Here's how the part is built. I have some questions about the finished solid (model axes, mm). A direction names the side the tool comes from. Give positions to 0.01 mm unless a question says otherwise; leave off trailing zeros. Loops run counter-clockwise (first coordinate to the right, second up) from the corner with the lowest first, then second, coordinate; pieces in that order, holes last.
Q1. I need wall thicknesses on line 1 (Y direction, x = 0, z = 5); line 2 (Z direction, x = 24, y = 40); line 3 (X direction, y = 9.5, z = 46). Which ranges of each line are inside material? Lowest first, please.
Q2. If we section it at B-B (z = 37.5): Please give me the cut outline in (x, y).
Q3. For faces 1 (the face through (3, 0, 0)), 2 (the face through (-2.75, -12.4, 25.04)), which set-ups out of +Z, -Z, +X, -X, +Y, -Y let a thin tool reach every point of the face, with its end or its side?
Q4. If we section it at C-C (x = 61): Please give me the cut outline in (y, z), plus the area to 3 significant figures.
Q5. If we section it at A-A (x = 8.5): Please give me the cut outline in (y, z), plus the area to 3 significant figures.
Q6. If we section it at D-D (x = 28): Please give me the cut outline in (y, z), plus the area to 3 significant figures.
Q7. Will these pins go through, and if not, where does the flat tip stop? P1, Ø10, axis at y = -5, z = 25, coming from the +X side; P2, Ø8, axis at x = -6, z = 33.5, coming from the +Y side; P3, Ø2, axis at x = -0.5, y = 0, coming from the -Z side; P4, Ø4, axis at x = 8, y = -45.5, coming from the -Z side.
from build123d import *

# Parameters (mm, degrees)
F0_R     = 12.7
F1_DEPTH = 50.8
F3_DEPTH = 2.54
F4_R     = 1.27
F5_DEPTH = 12.7


with BuildPart() as f1:
    # F0 (on Top) → F1 (new body)
    with BuildSketch(Plane.XY):
        Circle(F0_R)
    extrude(amount=F1_DEPTH)

    # F2 (on face) → F3 (join)
    with BuildSketch(Plane.XY.offset(50.8)):
        with BuildLine():
            Line((43.181052426, 26.7588622961), (25.5085228248, 43.9312561088))
            ThreePointArc((25.5085228248, 43.9312561088), (-43.9312561088, 25.5085228248), (-25.5085228248, -43.9312561088))
            Line((-25.5085228248, -43.9312561088), (-1.833987853, -50.7668837783))
            ThreePointArc((-1.833987853, -50.7668837783), (6.0769799698, -50.4352090751), (13.8403151675, -48.87827407))
            ThreePointArc((13.8403151675, -48.87827407), (5.917077838, -28.064349578), (10.982813992, -6.3771307669))
            ThreePointArc((10.982813992, -6.3771307669), (27.3066244447, 8.7731285653), (49.3108654889, 12.2097725094))
            ThreePointArc((49.3108654889, 12.2097725094), (46.8146101479, 19.7239011532), (43.181052426, 26.7588622961))
        make_face()
        with BuildLine():
            ThreePointArc((12.7, 0), (12.2631916257, -3.3021403894), (10.982813992, -6.3771307669))
            ThreePointArc((10.982813992, -6.3771307669), (-12.2631916257, 3.3021403894), (12.7, 0))
        make_face(mode=Mode.SUBTRACT)
        with BuildLine():
            ThreePointArc((63.0626482274, 7.4399192569), (56.4166545258, 10.4876551164), (49.3108654889, 12.2097725094))
            ThreePointArc((49.3108654889, 12.2097725094), (50.4263421578, 6.150123298), (50.8, 0))
            ThreePointArc((50.8, 0), (50.3191031963, -6.9733674448), (48.8855175779, -13.8147085071))
            ThreePointArc((48.8855175779, -13.8147085071), (54.5192002119, -18.4952896423), (56.6312561088, -25.5085228248))
            ThreePointArc((56.6312561088, -25.5085228248), (49.5659896786, -36.8900770946), (36.2312911329, -35.6080544659))
            ThreePointArc((36.2312911329, -35.6080544659), (25.9001181747, -43.7015317642), (13.8403151675, -48.87827407))
            ThreePointArc((13.8403151675, -48.87827407), (18.8584152746, -54.1958484669), (24.7998639903, -58.4569649064))
            ThreePointArc((24.7998639903, -58.4569649064), (62.9405164874, -58.5275782301), (82.0312561088, -25.5085228248))
            ThreePointArc((82.0312561088, -25.5085228248), (76.9503115141, -6.4992624462), (63.0626482274, 7.4399192569))
        make_face()
        with BuildLine():
            ThreePointArc((50.8, 0), (50.4263421578, 6.150123298), (49.3108654889, 12.2097725094))
            ThreePointArc((49.3108654889, 12.2097725094), (27.3066244447, 8.7731285653), (10.982813992, -6.3771307669))
            ThreePointArc((10.982813992, -6.3771307669), (5.917077838, -28.064349578), (13.8403151675, -48.87827407))
            ThreePointArc((13.8403151675, -48.87827407), (25.9001181747, -43.7015317642), (36.2312911329, -35.6080544659))
            ThreePointArc((36.2312911329, -35.6080544659), (32.9484420816, -19.1313921186), (48.8855175779, -13.8147085071))
            ThreePointArc((48.8855175779, -13.8147085071), (50.3191031963, -6.9733674448), (50.8, 0))
        make_face()
        with BuildLine():
            ThreePointArc((12.7, 0), (-12.2631916257, 3.3021403894), (10.982813992, -6.3771307669))
            ThreePointArc((10.982813992, -6.3771307669), (12.2631916257, -3.3021403894), (12.7, 0))
        make_face()
        with BuildLine():
            Line((63.0626482274, 7.4399192569), (43.181052426, 26.7588622961))
            ThreePointArc((43.181052426, 26.7588622961), (46.8146101479, 19.7239011532), (49.3108654889, 12.2097725094))
            ThreePointArc((49.3108654889, 12.2097725094), (56.4166545258, 10.4876551164), (63.0626482274, 7.4399192569))
        make_face()
        with BuildLine():
            ThreePointArc((13.8403151675, -48.87827407), (6.0769799698, -50.4352090751), (-1.833987853, -50.7668837783))
            Line((-1.833987853, -50.7668837783), (24.7998639903, -58.4569649064))
            ThreePointArc((24.7998639903, -58.4569649064), (18.8584152746, -54.1958484669), (13.8403151675, -48.87827407))
        make_face()
    extrude(amount=F3_DEPTH)

    # F4 (on face) → F5 (cut)
    with BuildSketch(Plane(origin=(0, 0, 0), x_dir=(1, 0, 0), z_dir=(0, 0, -1))):
        Circle(F4_R)
    extrude(amount=-F5_DEPTH, mode=Mode.SUBTRACT)


solid = f1.part
Check sheet entries:
1. line 1: y = -12.7 to -1.27, 1.27 to 12.7
1. line 2: z = 50.8 to 53.34
1. line 3: x = -8.43 to 8.43
2. outline: circle Ø25.4 at (0, 0)
3. face 1: -Z, +X, -X, +Y, -Y
3. face 2: -Z
4. outline: (-59.57, 50.8) - (9.44, 50.8) - (9.44, 53.34) - (-59.57, 53.34) - close
4. area: 175 mm2
5. outline: (-53.75, 50.8) - (-9.44, 50.8) - (-9.44, 0) - (9.44, 0) - (9.44, 50.8) - (50.08, 50.8) - (50.08, 53.34) - (-53.75, 53.34) - close
5. area: 1,220 mm2
6. outline: (-60.12, 50.8) - (41.51, 50.8) - (41.51, 53.34) - (-60.12, 53.34) - close
6. area: 258 mm2
7. P1: stops at x = 12.7
7. P2: stops at y = 12.54
7. P3: stops at z = 0
7. P4: stops at z = 50.8
